For this review, take the finished solid that the model builds, in its own axes (mm). A direction names the side the tool comes from. Round coordinates to 2 decimals unless told otherwise and drop trailing zeros. Write each loop counter-clockwise with the first axis right and the second up, starting at its lowest first coordinate (ties: lowest second). Pieces come first, ordered by that corner, then holes. Notation, with made-up numbers: (-26, 83.5) -> (11, 83.5) arc R14 cw to (11, 91.5) -> close; hole circle Ø7 at (-7, 47). An arc over 180 degrees is marked (long way). Answer as CSV lines item,"result". Start each with the question number.
Item 1: Wall thickness on probe 1 along Y at (x, z) = (6, 27); probe 2 along Z at (x, y) = (-27, 32.5); probe 3 along X at (y, z) = (-13.5, 19.5): over which ranges is each line inside the solid? List them lowest first. Write a range as from..to.
Item 2: For pin 1 Ø1.5 at (x, z) = (8.5, 22.5) entering from -Y; pin 2 Ø5 at (y, z) = (-8.5, 29) entering from -X; pin 3 Ø12.5 at (x, z) = (-2.5, 21.5) entering from +Y, all flat-tipped, find the tip position at first contact; note any pin that passes through.
Item 3: Take a section at C-C on z = 10.5. Give the boundary of the cut face in (x, y), then the cut area to 3 significant figures.
Item 4: Machinability: for faces 1 (the flat face through (22.225, 0, 20)), 2 (the flat face through (0, -15.352, 20)), 3 (the flat face through (0, 15.352, 20)), which of the approach directions +Z, -Z, +X, -X, +Y, -Y give a long, thin tool a straight path to every point of the face, cutting with its end or side? Answer none if there is none.
Item 5: Take a section at D-D on z = 3. Give the boundary of the cut face in (x, y), then the cut area to 3 significant figures.
Item 6: Take a section at A-A on x = 0. Give the boundary of the cut face in (y, z).
Item 7: Take a section at B-B on y = 0. Give the boundary of the cut face in (x, z).
```python
from build123d import *

# Parameters (mm, degrees)
F0_R     = 47.137845
F1_DEPTH = 7.61904
F2_R     = 3.146541
F4_W     = 44.450962
F4_H     = 30.703868
F5_DEPTH = 25.4


with BuildPart() as f1:
    # F0 (on Top) → F1 (new body)
    with BuildSketch(Plane.XY):
        Circle(F0_R)
    extrude(amount=F1_DEPTH)

    # F2
    f2_edges = [f1.edges().sort_by_distance(p)[0] for p in [
        (-47.137845, 0, 7.61904),
    ]]
    fillet(f2_edges, radius=F2_R)

    # F4 (on face) → F5 (join)
    with BuildSketch(Plane.XY.offset(7.61904)):
        Rectangle(F4_W, F4_H)
    extrude(amount=F5_DEPTH)


solid = f1.part
```
Output values:
1,probe 1,"y = -15.35..15.35"
1,probe 2,"z = 0..7.62"
1,probe 3,"x = -22.23..22.23"
2,pin 1,"stops at y = -15.35"
2,pin 2,"stops at x = -22.23"
2,pin 3,"stops at y = 15.35"
3,outline,"(-22.23, -15.35) -> (22.23, -15.35) -> (22.23, 15.35) -> (-22.23, 15.35) -> close"
3,area,"1,360 mm^2"
4,face 1,"+Z, +X, +Y, -Y"
4,face 2,"+Z, +X, -X, -Y"
4,face 3,"+Z, +X, -X, +Y"
5,outline,"circle Ø94.28 at (0, 0)"
5,area,"6,980 mm^2"
6,outline,"(-47.14, 0) -> (47.14, 0) -> (47.14, 4.47) arc R3.15 ccw to (43.99, 7.62) -> (15.35, 7.62) -> (15.35, 33.02) -> (-15.35, 33.02) -> (-15.35, 7.62) -> (-43.99, 7.62) arc R3.15 ccw to (-47.14, 4.47) -> close"
7,outline,"(-47.14, 0) -> (47.14, 0) -> (47.14, 4.47) arc R3.15 ccw to (43.99, 7.62) -> (22.23, 7.62) -> (22.23, 33.02) -> (-22.23, 33.02) -> (-22.23, 7.62) -> (-43.99, 7.62) arc R3.15 ccw to (-47.14, 4.47) -> close"
